```python
from build123d import *

# Parameters (mm, degrees)
SCHIZZO1_W                   = 558
SCHIZZO1_H                   = 441.5
ESTRUSIONE_ESTRUSIONE1_DEPTH = 6
SCHIZZO2_R                   = 2.25
TAGLIO_ESTRUSIONE1_DEPTH     = 10
TAGLIO_ESTRUSIONE2_DEPTH     = 10


with BuildPart() as part:
    # Schizzo1 → Estrusione-Estrusione1 (new body)
    with BuildSketch(Plane(origin=(0, 0, 0), x_dir=(1, 0, 0), z_dir=(0, 1, 0))):
        Rectangle(SCHIZZO1_W, SCHIZZO1_H)
    extrude(amount=ESTRUSIONE_ESTRUSIONE1_DEPTH)

    # Schizzo2 → Taglio-Estrusione1 (cut)
    with BuildSketch(Plane(origin=(0, 0, 0), x_dir=(-1, 0, 0), z_dir=(0, -1, 0))):
        with Locations(Location((-221, 207.25, 0), (0, 0, 90))):
            Circle(SCHIZZO2_R)
        with Locations(Location((-221, 188.75, 0), (0, 0, 90))):
            Circle(SCHIZZO2_R)
        with Locations(Location((-247, 162.75, 0), (0, 0, 90))):
            Circle(SCHIZZO2_R)
        with Locations(Location((-265.5, 162.75, 0), (0, 0, 90))):
            Circle(SCHIZZO2_R)
        with Locations(Location((221, 207.25, 0), (0, 0, 90))):
            Circle(SCHIZZO2_R)
        with Locations(Location((221, 188.75, 0), (0, 0, 90))):
            Circle(SCHIZZO2_R)
        with Locations(Location((247, 162.75, 0), (0, 0, 90))):
            Circle(SCHIZZO2_R)
        with Locations(Location((265.5, 162.75, 0), (0, 0, 90))):
            Circle(SCHIZZO2_R)
        with Locations(Location((265.5, -162.75, 0), (0, 0, 90))):
            Circle(SCHIZZO2_R)
        with Locations(Location((247, -162.75, 0), (0, 0, 90))):
            Circle(SCHIZZO2_R)
        with Locations(Location((-265.5, -162.75, 0), (0, 0, 90))):
            Circle(SCHIZZO2_R)
        with Locations(Location((-247, -162.75, 0), (0, 0, 90))):
            Circle(SCHIZZO2_R)
        with Locations(Location((-87.5, -195.25, 0), (0, 0, 90))):
            Circle(SCHIZZO2_R)
    extrude(amount=-TAGLIO_ESTRUSIONE1_DEPTH, mode=Mode.SUBTRACT)

    # Schizzo3 → Taglio-Estrusione2 (cut)
    with BuildSketch(Plane(origin=(0, 6, 0), x_dir=(1, 0, 0), z_dir=(0, 1, 0))):
        Polygon((-279, 0), (-261.3, 0), (-268.8, 10), (-233.4, 10), (-240.9, 0), (-223.2, 0), (-205.5, 0), (-213, 10), (-177.6, 10), (-185.1, 0), (-167.4, 0), (-149.7, 0), (-157.2, 10), (-121.8, 10), (-129.3, 0), (-111.6, 0), (-93.9, 0), (-101.4, 10), (-66, 10), (-73.5, 0), (-55.8, 0), (-38.1, 0), (-45.6, 10), (-10.2, 10), (-17.7, 0), (0, 0), (17.7, 0), (10.2, 10), (45.6, 10), (38.1, 0), (55.8, 0), (73.5, 0), (66, 10), (101.4, 10), (93.9, 0), (111.6, 0), (129.3, 0), (121.8, 10), (157.2, 10), (149.7, 0), (167.4, 0), (185.1, 0), (177.6, 10), (213, 10), (205.5, 0), (223.2, 0), (240.9, 0), (233.4, 10), (268.8, 10), (261.3, 0), (279, 0), (279, -220.75), (-279, -220.75), align=None)
    extrude(amount=-TAGLIO_ESTRUSIONE2_DEPTH, mode=Mode.SUBTRACT)


solid = part.part
```
CAD build for the part. Positions are in the model's coordinates, mm. Coordinates: 2 decimals unless noted, no trailing zeros.
(1) Saw through at A-A, the plane y = 2.35. Count the separate pieces of the cut face and the enclosed holes in it, and give its area (3 significant figures).
Solution:
separate pieces: 1
enclosed holes: 8
area: 120,000 mm2
(2) Drill centre lines: L1, parallel to X at y = 4.55, z = -207.25; L2, parallel to X at y = 4.45, z = -162.75; L3, parallel to Z at x = -221, y = 2.4. Where is each one in solid material? Low to high.
Solution:
L1: x = -279 to -223.25, -218.75 to 218.75, 223.25 to 279
L2: x = -279 to -267.75, -263.25 to -249.25, -244.75 to 244.75, 249.25 to 263.25, 267.75 to 279
L3: z = -220.75 to -209.5, -205 to -191, -186.5 to 0
(3) Pin check, flat tips, straight feed: pin 1 Ø3 at (x, y) = (-141, 3.5) entering from +Z; pin 2 Ø3.5 at (x, z) = (221, -188.75) entering from +Y. Stop position of each tip, or through.
Solution:
pin 1: stops at z = -10
pin 2: passes through
